```python
from build123d import *

# Parameters (mm, degrees)
F1_DEPTH  = 215
F2_SIZE   = 10
F3_R      = 20
F3_R_2    = 30
F4_DEPTH  = 8
F5_R      = 15
F5_R_2    = 25
F6_DEPTH  = 5
F7_R      = 4.99999
F8_R      = 15
F8_R_2    = 7.5
F9_DEPTH  = 5
F10_W     = 89
F10_H     = 199
F11_DEPTH = 10
F12_W     = 46
F12_H     = 16
F12_R     = 4
F13_DEPTH = 10
F14_W     = 70
F14_H     = 70
F14_W_2   = 60
F14_H_2   = 60
F14_R     = 7.5
F15_DEPTH = 10


# Not quite as in the source:
# - a fillet or chamfer is up to 0.001 mm smaller than in the source, because OpenCascade refuses the exact size


with BuildPart() as f1:
    # F0 (on Top) → F1 (new body)
    with BuildSketch(Plane.XY):
        Polygon((0, 110), (0, 0), (105, 0), (105, 110), (95, 120), (10, 120), align=None)
    extrude(amount=F1_DEPTH)

    # F2
    f2_edges = [f1.edges().sort_by_distance(p)[0] for p in [
        (52.5, 120, 215),
        (52.5, 120, 0),
    ]]
    chamfer(f2_edges, length=F2_SIZE)

    # F3 (on face) → F4 (cut)
    with BuildSketch(Plane(origin=(0, 120, 0), x_dir=(-1, 0, 0), z_dir=(0, 1, 0))):
        with Locations((-52.5, 150)):
            Circle(F3_R)
        with Locations((-52.5, 70)):
            Circle(F3_R_2)
    extrude(amount=-F4_DEPTH, mode=Mode.SUBTRACT)

    # F5 (on face) → F6 (join)
    with BuildSketch(Plane(origin=(0, 112, 0), x_dir=(-1, 0, 0), z_dir=(0, 1, 0))):
        with Locations((-52.5, 150)):
            Circle(F5_R)
        with Locations((-52.5, 70)):
            Circle(F5_R_2)
    extrude(amount=F6_DEPTH)

    # F7 (radius 5 in the source; OpenCascade refuses exactly that, so slightly less here)
    f7_edges = [f1.edges().sort_by_distance(p)[0] for p in [
        (77.5, 117, 70),
        (67.5, 117, 150),
    ]]
    fillet(f7_edges, radius=F7_R)

    # F8 (on face) → F9 (cut)
    with BuildSketch(Plane(origin=(0, 117, 0), x_dir=(-1, 0, 0), z_dir=(0, 1, 0))):
        with Locations((-52.5, 70)):
            Circle(F8_R)
        with Locations((-52.5, 70)):
            Circle(F8_R_2, mode=Mode.SUBTRACT)
    extrude(amount=-F9_DEPTH, mode=Mode.SUBTRACT)

    # F10 (on face) → F11 (cut)
    with BuildSketch(Plane.XZ):
        with Locations((52.5, 107.5)):
            Rectangle(F10_W, F10_H)
    extrude(amount=-F11_DEPTH, mode=Mode.SUBTRACT)

    # F12 (on face) → F13 (join)
    with BuildSketch(Plane.XZ.offset(-10)):
        with Locations((52.5, 189)):
            Rectangle(F12_W, F12_H)
        with Locations((39.5, 191)):
            Circle(F12_R, mode=Mode.SUBTRACT)
        with Locations((65.5, 191)):
            Circle(F12_R, mode=Mode.SUBTRACT)
    extrude(amount=F13_DEPTH)

    # F14 (on face) → F15 (join)
    with BuildSketch(Plane.XZ.offset(-10)):
        with Locations((52.5, 60)):
            Rectangle(F14_W, F14_H)
        with Locations((52.5, 60)):
            Rectangle(F14_W_2, F14_H_2, mode=Mode.SUBTRACT)
        with Locations((67.5, 55)):
            Circle(F14_R)
        with Locations((37.5, 55)):
            Circle(F14_R)
    extrude(amount=F15_DEPTH)


solid = f1.part
```
For this review, take the finished solid that the model builds, in its own axes (mm). A direction names the side the tool comes from. Give positions to 0.01 mm unless a question says otherwise; leave off trailing zeros.
Item 1: Wall thickness on probe 1 along Y at (x, z) = (67, 190); probe 2 along Y at (x, z) = (37, 91); probe 3 along Z at (x, y) = (16.5, 112.5): over which ranges is each line inside the solid? List them lowest first.
Item 2: Insertion check: P1, Ø20, axis at x = 49, z = 146, coming from the +Y side; P2, Ø2, axis at x = 45, z = 188, coming from the -Y side; P3, Ø6.5, axis at x = 39, z = 190.5, coming from the -Y side; P4, Ø4, axis at x = 29.5, z = 58, coming from the +Y side. Each pin has a flat end and moves straight along its axis. Give the tip position at first contact, or say it passes through.
Item 3: The part is to be moulded in two halves that separate along Z. For faces 4 (the face through (87.5, 5, 60)), 5 (the face through (53, 120, 106)), say which applies: +Z half, -Z half, draft (parallel to the pull), parting line (faces both ways), or undercut.
Item 4: Machinability: for faces 1 (the face through (52, 5, 95)), 2 (the face through (0, 56, 106)), 3 (the face through (74.611, 116.056, 90.275)), which of the approach directions +Z, -Z, +X, -X, +Y, -Y give a long, thin tool a straight path to every point of the face, cutting with its end or side? Answer none if there is none.
Established:
1. probe 1: y = 10 to 120
1. probe 2: y = 0 to 112
1. probe 3: z = 2.5 to 212.5
2. P1: stops at y = 117
2. P2: stops at y = 0
2. P3: stops at y = 10
2. P4: stops at y = 115.08
3. face 4: undercut
3. face 5: draft
4. face 1: -Y
4. face 2: +Z, -Z, -X, +Y, -Y
4. face 3: +Y
